Work out the finished part from the listing and answer in its coordinate system (mm). Coordinates: 2 decimals unless noted, no trailing zeros. Order: outer loops, then holes, each group sorted by start corner. A loop starts at its lowest first (then second) coordinate and runs counter-clockwise, first axis right, second up. Notation, with made-up numbers: (82.5, 34.25) - (139.5, 34.25) arc R21 ccw to (139.5, 50.25) - close; hole circle Ø4 at (-21, -11.75). An arc over 180 degrees is marked (long way). Use CSV: the item, a comma, the result in double quotes. Start each with the question number.
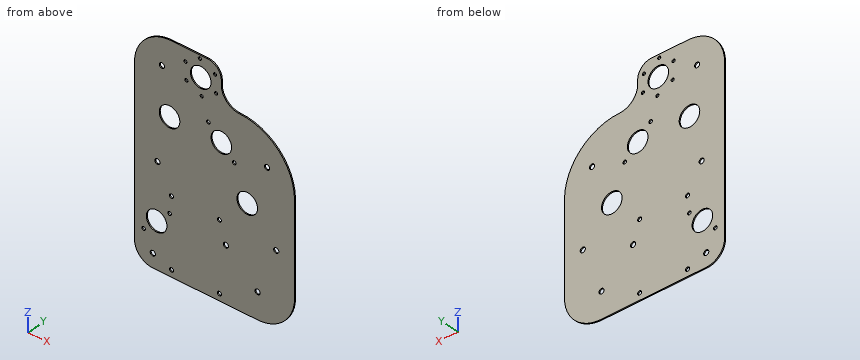
from build123d import *

# Parameters (mm, degrees)
SKETCH1_W               = 222.123
SKETCH1_H               = 254.783638074
SKETCH1_R               = 14.2875
SKETCH1_R_2             = 1.27
BOSS_EXTRUDE1_DEPTH     = 1.5875
F_10_CLEARANCE_HOLE1_D  = 4.9784
SKETCH4_R               = 2.8067
CUT_EXTRUDE1_DEPTH      = 170.014355888
SKETCH5_R               = 1.5875
CUT_EXTRUDE2_DEPTH      = 170.014355888
SKETCH6_W               = 222.123
SKETCH6_H               = 1.5875
BOSS_EXTRUDE2_DEPTH     = 50.8
SKETCH7_W               = 101.6
SKETCH7_H               = 50.8
CUT_EXTRUDE3_DEPTH      = 210.975001632
SKETCH8_R               = 14.2875
CUT_EXTRUDE5_DEPTH      = 210.975001632
SKETCH9_R               = 2.15
CUT_EXTRUDE6_DEPTH      = 210.975001632
SKETCH10_R              = 14.2875
SKETCH10_R_2            = 1.27
CUT_EXTRUDE7_DEPTH      = 210.975001632
F_10_CLEARANCE_HOLE2_D  = 4.9784
CUT_EXTRUDE8_DEPTH      = 210.975001632
CUT_EXTRUDE9_DEPTH      = 210.975001632
FILLET1_R               = 25.4
CUT_EXTRUDE10_DEPTH     = 210.975001632
CUT_EXTRUDE11_DEPTH     = 210.975001632
CUT_EXTRUDE13_DEPTH     = 210.975001632
SKETCH18_R              = 1.27
CUT_EXTRUDE14_DEPTH     = 210.975001632
F_1_4_CLEARANCE_HOLE1_D = 7.14248


with BuildPart() as part:
    # Sketch1 → Boss-Extrude1 (new body)
    with BuildSketch(Plane(origin=(0, 0, 0), x_dir=(1, 0, 0), z_dir=(0, 1, 0))):
        Rectangle(SKETCH1_W, SKETCH1_H)
        with Locations(Location((9.4615, -78.750819037, 0), (0, 0, 270))):
            Circle(SKETCH1_R, mode=Mode.SUBTRACT)
        with Locations(Location((45.4025, -16.499180963, 0), (0, 0, 270))):
            Circle(SKETCH1_R, mode=Mode.SUBTRACT)
        with Locations(Location((-62.4205, -78.750819037, 0), (0, 0, 270))):
            Circle(SKETCH1_R, mode=Mode.SUBTRACT)
        with Locations(Location((-8.499012242, -96.71133128, 0), (0, 0, 270))):
            Circle(SKETCH1_R_2, mode=Mode.SUBTRACT)
        with Locations(Location((27.422012242, -60.790306795, 0), (0, 0, 270))):
            Circle(SKETCH1_R_2, mode=Mode.SUBTRACT)
    extrude(amount=BOSS_EXTRUDE1_DEPTH)

    # #10 Clearance Hole1 (through all)
    with Locations(Plane(origin=(0, 1.5875, 0), x_dir=(1, 0, 0), z_dir=(0, 1, 0))):
        with Locations((-8.499012242, -96.71133128), (27.422012242, -60.790306795)):
            Hole(F_10_CLEARANCE_HOLE1_D / 2)

    # Sketch4 → Cut-Extrude1 (cut, through all)
    with BuildSketch(Plane(origin=(0, 0, 0), x_dir=(-1, 0, 0), z_dir=(0, -1, 0))):
        with Locations(Location((59.692539866, 117.866819037, 0), (0, 0, 90))):
            Circle(SKETCH4_R)
        with Locations(Location((59.692539866, 22.616819037, 0), (0, 0, 90))):
            Circle(SKETCH4_R)
        with Locations(Location((-6.733539866, 117.866819037, 0), (0, 0, 90))):
            Circle(SKETCH4_R)
        with Locations(Location((-6.733539866, 22.616819037, 0), (0, 0, 90))):
            Circle(SKETCH4_R)
    extrude(amount=-CUT_EXTRUDE1_DEPTH, mode=Mode.SUBTRACT)

    # Sketch5 → Cut-Extrude2 (cut, through all)
    with BuildSketch(Plane.XZ):
        with Locations(Location((59.770116522, -91.195174152, 0), (0, 0, 270))):
            Circle(SKETCH5_R)
    extrude(amount=-CUT_EXTRUDE2_DEPTH, mode=Mode.SUBTRACT)

    # Sketch6 → Boss-Extrude2 (add)
    with BuildSketch(Plane.XY.offset(127.391819037)):
        with Locations((0, 0.79375)):
            Rectangle(SKETCH6_W, SKETCH6_H)
    extrude(amount=BOSS_EXTRUDE2_DEPTH)

    # Sketch7 → Cut-Extrude3 (cut, through all)
    with BuildSketch(Plane(origin=(0, 0, 0), x_dir=(-1, 0, 0), z_dir=(0, -1, 0))):
        with Locations((-60.2615, -152.791819037)):
            Rectangle(SKETCH7_W, SKETCH7_H)
    extrude(amount=-CUT_EXTRUDE3_DEPTH, mode=Mode.SUBTRACT)

    # Sketch8 → Cut-Extrude5 (cut, through all)
    with BuildSketch(Plane(origin=(0, 1.5875, 0), x_dir=(1, 0, 0), z_dir=(0, 1, 0))):
        with Locations(Location((-19.1135, -149.616819037, 0), (0, 0, 270))):
            Circle(SKETCH8_R)
    extrude(amount=-CUT_EXTRUDE5_DEPTH, mode=Mode.SUBTRACT)

    # Sketch9 → Cut-Extrude6 (cut, through all)
    with BuildSketch(Plane(origin=(0, 1.5875, 0), x_dir=(1, 0, 0), z_dir=(0, 1, 0))):
        with Locations(Location((-17.801836865, -125.840471629, 0), (0, 0, 270))):
            Circle(SKETCH9_R)
        with Locations(Location((2.133252432, -138.86457893, 0), (0, 0, 270))):
            Circle(SKETCH9_R)
        with Locations(Location((0.821589297, -162.640926338, 0), (0, 0, 270))):
            Circle(SKETCH9_R)
        with Locations(Location((-20.425163135, -173.393166445, 0), (0, 0, 270))):
            Circle(SKETCH9_R)
        with Locations(Location((-40.360252432, -160.369059145, 0), (0, 0, 270))):
            Circle(SKETCH9_R)
        with Locations(Location((-39.048589297, -136.592711737, 0), (0, 0, 270))):
            Circle(SKETCH9_R)
    extrude(amount=-CUT_EXTRUDE6_DEPTH, mode=Mode.SUBTRACT)

    # Sketch10 → Cut-Extrude7 (cut, through all)
    with BuildSketch(Plane(origin=(0, 0, 0), x_dir=(-1, 0, 0), z_dir=(0, -1, 0))):
        with Locations(Location((80.318324186, 64.242728022, 0), (0, 0, 90))):
            Circle(SKETCH10_R)
        with Locations(Location((62.357811944, 46.28221578, 0), (0, 0, 90))):
            Circle(SKETCH10_R_2)
        with Locations(Location((98.278836428, 82.203240264, 0), (0, 0, 90))):
            Circle(SKETCH10_R_2)
    extrude(amount=-CUT_EXTRUDE7_DEPTH, mode=Mode.SUBTRACT)

    # #10 Clearance Hole2 (through all)
    with Locations(Plane(origin=(0, 0, 0), x_dir=(-1, 0, 0), z_dir=(0, -1, 0))):
        with Locations((98.278836428, 82.203240264), (62.357811944, 46.28221578)):
            Hole(F_10_CLEARANCE_HOLE2_D / 2)

    # Sketch13 → Cut-Extrude8 (cut, through all)
    with BuildSketch(Plane(origin=(0, 1.5875, 0), x_dir=(1, 0, 0), z_dir=(0, 1, 0))):
        with BuildLine():
            Line((60.2615, 127.391819037), (111.0615, 127.391819037))
            Line((111.0615, 127.391819037), (111.0615, 76.591819037))
            ThreePointArc((111.0615, 76.591819037), (96.182524484, 112.512843522), (60.2615, 127.391819037))
        make_face()
    extrude(amount=-CUT_EXTRUDE8_DEPTH, mode=Mode.SUBTRACT)

    # Sketch14 → Cut-Extrude9 (cut, through all)
    with BuildSketch(Plane(origin=(0, 1.5875, 0), x_dir=(1, 0, 0), z_dir=(0, 1, 0))):
        with BuildLine():
            Line((34.8615, -127.391819037), (111.0615, -127.391819037))
            Line((111.0615, -127.391819037), (111.0615, -51.191819037))
            ThreePointArc((111.0615, -51.191819037), (88.743036726, -105.073355764), (34.8615, -127.391819037))
        make_face()
    extrude(amount=-CUT_EXTRUDE9_DEPTH, mode=Mode.SUBTRACT)

    # Fillet1
    fillet1_edges = [part.edges().sort_by_distance(p)[0] for p in [
        (9.4615, 0.79375, 127.391819037),
    ]]
    fillet(fillet1_edges, radius=FILLET1_R - 0.0001)  # a hair under: the kernel refuses the full size

    # Sketch15 → Cut-Extrude10 (cut, through all)
    with BuildSketch(Plane(origin=(0, 1.5875, 0), x_dir=(1, 0, 0), z_dir=(0, 1, 0))):
        with BuildLine():
            Line((-111.0615, 101.991819037), (-111.0615, 127.391819037))
            Line((-111.0615, 127.391819037), (-85.6615, 127.391819037))
            ThreePointArc((-85.6615, 127.391819037), (-103.622012242, 119.95233128), (-111.0615, 101.991819037))
        make_face()
    extrude(amount=-CUT_EXTRUDE10_DEPTH, mode=Mode.SUBTRACT)

    # Sketch16 → Cut-Extrude11 (cut, through all)
    with BuildSketch(Plane(origin=(0, 1.5875, 0), x_dir=(1, 0, 0), z_dir=(0, 1, 0))):
        with BuildLine():
            Line((-111.0615, -127.391819037), (-111.0615, -178.191819037))
            Line((-111.0615, -178.191819037), (-60.2615, -178.191819037))
            ThreePointArc((-60.2615, -178.191819037), (-96.182524484, -163.312843522), (-111.0615, -127.391819037))
        make_face()
    extrude(amount=-CUT_EXTRUDE11_DEPTH, mode=Mode.SUBTRACT)

    # Sketch17 → Cut-Extrude13 (cut, through all)
    with BuildSketch(Plane(origin=(0, 1.5875, 0), x_dir=(1, 0, 0), z_dir=(0, 1, 0))):
        with BuildLine():
            Line((9.4615, -178.191819037), (9.4615, -159.141819037))
            ThreePointArc((9.4615, -159.141819037), (3.881884182, -172.612203219), (-9.5885, -178.191819037))
            Line((-9.5885, -178.191819037), (9.4615, -178.191819037))
        make_face()
    extrude(amount=-CUT_EXTRUDE13_DEPTH, mode=Mode.SUBTRACT)

    # Sketch18 → Cut-Extrude14 (cut, through all)
    with BuildSketch(Plane(origin=(0, 1.5875, 0), x_dir=(1, 0, 0), z_dir=(0, 1, 0))):
        with Locations(Location((72.9615, -75.808180963, 0), (0, 0, 270))):
            Circle(SKETCH18_R)
        with Locations(Location((85.6615, 25.791819037, 0), (0, 0, 270))):
            Circle(SKETCH18_R)
        with Locations(Location((15.8115, 51.191819037, 0), (0, 0, 270))):
            Circle(SKETCH18_R)
        with Locations(Location((-85.6615, 108.341819037, 0), (0, 0, 270))):
            Circle(SKETCH18_R)
        with Locations(Location((-79.3115, -13.091819037, 0), (0, 0, 270))):
            Circle(SKETCH18_R)
        with Locations(Location((-72.9615, -140.091819037, 0), (0, 0, 270))):
            Circle(SKETCH18_R)
    extrude(amount=-CUT_EXTRUDE14_DEPTH, mode=Mode.SUBTRACT)

    # 1/4 Clearance Hole1 (through all)
    with Locations(Plane(origin=(0, 1.5875, 0), x_dir=(1, 0, 0), z_dir=(0, 1, 0))):
        with Locations((-72.9615, -140.091819037), (72.9615, -75.808180963), (85.6615, 25.791819037), (15.8115, 51.191819037), (59.770116522, 91.195174152), (-79.3115, -13.091819037), (-85.6615, 108.341819037)):
            Hole(F_1_4_CLEARANCE_HOLE1_D / 2)


solid = part.part
1) The part is cut by section D-D on z = 111. Determine the outline of the cut face in (x, y), plus the area to 3 significant figures.
2) The part is cut by section B-B on z = -71. Determine the outline of the cut face in (x, y), plus the area to 3 significant figures.
3) The part is cut by section C-C on y = 1.2. State how many separate pieces and enclosed holes the cut face has, plus the area to 3 significant figures.
4) The part is cut by section A-A on x = 73. Determine the outline of the cut face in (y, z).
5) Straight lines are drawn through the part: line 1 (Z direction, x = -41, y = 1.5); line 2 (Z direction, x = -72, y = 1); line 3 (Z direction, x = 19, y = 0.15). For each, find the intervals that lie inside material, in ascending order. Write a range as [from, to].
Answer key:
1,outline,"(-111.06, 0) - (82.08, 0) - (82.08, 1.59) - (-111.06, 1.59) - close"
1,area,"307 mm^2"
2,outline,"(-111.06, 0) - (-92.91, 0) - (-92.91, 1.59) - (-111.06, 1.59) - close; (-67.73, 0) - (111.06, 0) - (111.06, 1.59) - (-67.73, 1.59) - close"
2,area,"313 mm^2"
3,separate pieces,"1"
3,enclosed holes,"26"
3,area,"56,500 mm^2"
4,outline,"(0, -125.77) - (1.59, -125.77) - (1.59, 72.24) - (0, 72.24) - close; (0, 79.38) - (1.59, 79.38) - (1.59, 117.16) - (0, 117.16) - close"
5,line 1,"[-127.39, 135.69], [137.5, 158.32], [162.42, 178.19]"
5,line 2,"[-127.39, -75.86], [-52.63, 68.15], [89.35, 136.65], [143.53, 176.82]"
5,line 3,"[-127.39, -52.8], [-49.58, 68.11], [89.39, 132.95]"
